```python
from build123d import *

# Parameters (mm, degrees)
SKETCH1_W           = 41
SKETCH1_H           = 41
BOSS_EXTRUDE1_DEPTH = 640
SKETCH2_W           = 47
SKETCH2_H           = 47
BOSS_EXTRUDE2_DEPTH = 20
SKETCH3_W           = 600
SKETCH3_H           = 31
CUT_EXTRUDE1_DEPTH  = 10


with BuildPart() as part:
    # Sketch1 → Boss-Extrude1 (new body)
    with BuildSketch(Plane.XY):
        Rectangle(SKETCH1_W, SKETCH1_H)
    extrude(amount=BOSS_EXTRUDE1_DEPTH)

    # Sketch2 → Boss-Extrude2 (add)
    with BuildSketch(Plane(origin=(0, 0, 0), x_dir=(-1, 0, 0), z_dir=(0, 0, -1))):
        Rectangle(SKETCH2_W, SKETCH2_H)
    boss_extrude2 = extrude(amount=-BOSS_EXTRUDE2_DEPTH)

    # Mirror1: Boss-Extrude2 across plane
    add(boss_extrude2.mirror(Plane(origin=(0, 0, 320), x_dir=(1, 0, 0), z_dir=(0, 0, -1))))

    # Sketch3 → Cut-Extrude1 (cut)
    with BuildSketch(Plane(origin=(20.5, 0, 0), x_dir=(0, 0, -1), z_dir=(1, 0, 0))):
        with Locations((-320, 0)):
            Rectangle(SKETCH3_W, SKETCH3_H)
    extrude(amount=-CUT_EXTRUDE1_DEPTH, mode=Mode.SUBTRACT)


solid = part.part
```
Design review of the part built by this model. Coordinates are the model's own, in mm. A direction names the side the tool comes from. Coordinates: 2 decimals unless noted, no trailing zeros. Order: outer loops, then holes, each group sorted by start corner. A loop starts at its lowest first (then second) coordinate and runs counter-clockwise, first axis right, second up. Notation, with made-up numbers: (36, 13.25) -> (71, 13.25) arc R13 ccw to (71, 27.25) -> close; hole circle Ø9 at (19.5, -18). An arc over 180 degrees is marked (long way). One line per item, written item: value. Start each with the question number.
Q1. Insertion check: pin 1 Ø5 at (y, z) = (9, 459) entering from +X; pin 2 Ø1 at (x, z) = (-16.5, 75.5) entering from -Y; pin 3 Ø3 at (y, z) = (-16, 187) entering from +X. Each pin has a flat end and moves straight along its axis. Give the tip position at first contact, or say it passes through.
Q2. For probe 1 along Z at (x, y) = (18.5, -2.5); probe 2 along Y at (x, z) = (11, 355); probe 3 along Y at (x, z) = (9.5, 228), list the stretches that pass through material, from the lowest coordinate up.
Q3. Mouldability with a two-part tool opening along Y and no side actions: class faces 5 (the flat face through (0, 23.5, 630)), 6 (the flat face through (16, -15.5, 324)), 7 (the flat face through (-20.5, 0, 316)) as pulls with the +Y half, pulls with the -Y half, needs draft (parallel to the pull), parting line crosses it, or undercut.
Q4. Tool access review of faces 1 (the flat face through (16, 15.5, 324)), 2 (the flat face through (11, 0, 20)), 3 (the flat face through (0, 20.5, 316)), 4 (the flat face through (0, -20.5, 316)): name each direction out of +Z, -Z, +X, -X, +Y, -Y from which nothing blocks a thin tool from reaching the whole face with its end or side.
Q5. Take a section at B-B, the plane x = 3. State the section outline as (y, z) points, then the cut area to 3 significant figures.
Q6. Take a section at C-C, the plane z = 118. State the section outline as (x, y) points.
Q7. Take a section at A-A, the plane y = 8.5. State the section outline as (x, z) points.
Values follow:
1. pin 1: stops at x = 10.5
1. pin 2: stops at y = -20.5
1. pin 3: stops at x = 20.5
2. probe 1: z = 0 to 20, 620 to 640
2. probe 2: y = -20.5 to -15.5, 15.5 to 20.5
2. probe 3: y = -20.5 to 20.5
3. face 5: pulls with the +Y half
3. face 6: undercut
3. face 7: needs draft
4. face 1: +X
4. face 2: none
4. face 3: +X, -X, +Y
4. face 4: +X, -X, -Y
5. outline: (-23.5, 0) -> (23.5, 0) -> (23.5, 20) -> (20.5, 20) -> (20.5, 620) -> (23.5, 620) -> (23.5, 640) -> (-23.5, 640) -> (-23.5, 620) -> (-20.5, 620) -> (-20.5, 20) -> (-23.5, 20) -> close
5. area: 26,500 mm2
6. outline: (-20.5, -20.5) -> (20.5, -20.5) -> (20.5, -15.5) -> (10.5, -15.5) -> (10.5, 15.5) -> (20.5, 15.5) -> (20.5, 20.5) -> (-20.5, 20.5) -> close
7. outline: (-23.5, 0) -> (23.5, 0) -> (23.5, 20) -> (10.5, 20) -> (10.5, 620) -> (23.5, 620) -> (23.5, 640) -> (-23.5, 640) -> (-23.5, 620) -> (-20.5, 620) -> (-20.5, 20) -> (-23.5, 20) -> close
